Can you work these out from the model? Positions are in its coordinate system, mm. A direction names the side the tool comes from. Give positions to 0.01 mm unless a question says otherwise; leave off trailing zeros. Loops run counter-clockwise (first coordinate to the right, second up) from the corner with the lowest first, then second, coordinate; pieces in that order, holes last. Notation, with made-up numbers: (14, -29.75) - (39, -29.75) arc R28 cw to (39, -6.75) - close; hole circle Ø4 at (-37.75, -16). An arc over 180 degrees is marked (long way). Answer as a JSON object with one key per item and string values. Group by question number.
Item 1: Suppose I cut it at B-B on y = -12.5. Write out the boundary of the cut face in (x, z).
Item 2: Please list where these lines run through material, in increasing order: L1, parallel to Y at x = 1.5, z = 10.5; L2, parallel to X at y = -8, z = 5.75; L3, parallel to Z at x = 0, y = -9.
Item 3: Suppose I cut it at C-C on x = -14. Write out the boundary of the cut face in (y, z), and give its area (3 significant figures).
Item 4: Suppose I cut it at A-A on z = 8.5. Write out the boundary of the cut face in (x, y).
Item 5: Which directions (+Z, -Z, +X, -X, +Y, -Y) give clear straight access to the entire face, cutting with the end or side of a thin tool? Please do faces 4 (the flat face through (0, 20, 6)), 5 (the flat face through (3.5, -8, 7)).
Item 6: Suppose I cut it at D-D on y = 16. Write out the boundary of the cut face in (x, z), and give its area (3 significant figures).
Item 7: Thinking about a two-plate mould opening in X: for faces 1 (the flat face through (15, 15, 6)), 2 (the flat face through (-3.5, -8, 7)), 3 (the cylindrical face through (-9.89, 19.69, 6.34)), which applies, pulls with the +X half, pulls with the -X half, needs draft (parallel to the pull), parting line crosses it, or undercut?
Item 8: Will this pin go through, and if not, where does the flat tip stop? pin 1 (3 mm diameter, centred on y = 13.5, z = 5.5, fed in from -X).
from build123d import *

# Parameters (mm, degrees)
SKETCH1_W           = 38
SKETCH1_H           = 40
BOSS_EXTRUDE1_DEPTH = 12.5
SKETCH2_W           = 7
SKETCH2_H           = 16
CUT_EXTRUDE1_DEPTH  = 12
CHAMFER1_SIZE       = 9
FILLET1_R           = 4


with BuildPart() as part:
    # Sketch1 → Boss-Extrude1 (new body)
    with BuildSketch(Plane.XY):
        Rectangle(SKETCH1_W, SKETCH1_H)
    extrude(amount=BOSS_EXTRUDE1_DEPTH)

    # Sketch2 → Cut-Extrude1 (cut)
    with BuildSketch(Plane.XY.offset(12.5)):
        with Locations((0, -8)):
            Rectangle(SKETCH2_W, SKETCH2_H)
    extrude(amount=-CUT_EXTRUDE1_DEPTH, mode=Mode.SUBTRACT)

    # Chamfer1
    chamfer1_edges = [part.edges().sort_by_distance(p)[0] for p in [
        (-19, 20, 6.25),
        (19, 20, 6.25),
    ]]
    chamfer(chamfer1_edges, length=CHAMFER1_SIZE)

    # Fillet1
    fillet1_edges = [part.edges().sort_by_distance(p)[0] for p in [
        (-10, 20, 6.25),
        (10, 20, 6.25),
        (19, 11, 6.25),
        (-19, 11, 6.25),
        (19, -20, 6.25),
        (-19, -20, 6.25),
    ]]
    fillet(fillet1_edges, radius=FILLET1_R)


solid = part.part
Worked out:
{
 "1": {"outline": "(-19, 0) - (19, 0) - (19, 12.5) - (3.5, 12.5) - (3.5, 0.5) - (-3.5, 0.5) - (-3.5, 12.5) - (-19, 12.5) - close"},
 "2": {"L1": "y = -20 to -16, 0 to 20", "L2": "x = -19 to -3.5, 3.5 to 19", "L3": "z = 0 to 0.5"},
 "3": {"outline": "(-20, 0) - (16, 0) - (16, 12.5) - (-20, 12.5) - close", "area": "450 mm2"},
 "4": {"outline": "(-19, -16) arc R4 ccw to (-15, -20) - (15, -20) arc R4 ccw to (19, -16) - (19, 9.34) arc R4 ccw to (17.83, 12.17) - (11.17, 18.83) arc R4 ccw to (8.34, 20) - (-8.34, 20) arc R4 ccw to (-11.17, 18.83) - (-17.83, 12.17) arc R4 ccw to (-19, 9.34) - close; hole (-3.5, -16) - (3.5, -16) - (3.5, 0) - (-3.5, 0) - close"},
 "5": {"face 4": "+Z, -Z, +X, -X, +Y", "face 5": "+Z"},
 "6": {"outline": "(-14, 0) - (14, 0) - (14, 12.5) - (-14, 12.5) - close", "area": "350 mm2"},
 "7": {"face 1": "pulls with the +X half", "face 2": "undercut", "face 3": "pulls with the -X half"},
 "8": {"pin 1": "stops at x = -17.99"}
}
